```python
from build123d import *

# Parameters (mm, degrees)
F0_R      = 156.7807212082
F2_DEPTH  = 723.103761673
F4_DEPTH  = 289.7283732891
F5_DEPTH  = 25.4
F5_FACE_R = 156.7807212082


with BuildPart() as f2:
    # F0 (on Top) → F2 (new body)
    with BuildSketch(Plane.XY):
        Circle(F0_R)
    extrude(amount=F2_DEPTH)

    # F4 (add): a face of the model
    f4_faces = [f2.faces().sort_by_distance(p)[0] for p in [
        (0, 0, 0),
    ]]
    extrude(f4_faces, amount=F4_DEPTH)

    # F5 (add): a face of the model
    f5_faces = [f2.faces().sort_by_distance(p)[0] for p in [
        (0, 0, -289.7283732891),
    ]]
    extrude(f5_faces, amount=F5_DEPTH)

    # F5_face (on face) → F6 section 0
    with BuildSketch(Plane(origin=(0, 0, -315.1283732891), x_dir=(1, 0, 0), z_dir=(0, 0, -1)), mode=Mode.PRIVATE) as f6_s0:
        Circle(F5_FACE_R)
    loft([f6_s0.sketch, Vertex(0, 0, -691.5580034256)])


solid = f2.part
```
Geometry check sheet. Reference: the model listing, model coordinates, mm. Give positions to 0.01 mm unless a question says otherwise; leave off trailing zeros. Loops run counter-clockwise (first coordinate to the right, second up) from the corner with the lowest first, then second, coordinate; pieces in that order, holes last. Notation, with made-up numbers: M 64,74 L 80,74 A19 ccw 80,111 Z; hole C 64,20 d8. An arc over 180 degrees is marked long. Answer as CSV lines item,"result".
Item 1: Cross-section at B-B on z = -486.5. Record the cut outline in (x, y).
Values:
outline,"C 0,0 d170.81"
Item 2: Depth check by flat-ended pin: P1, Ø1.5, axis at y = -85, z = 559.5, coming from the -X side; P2, Ø3, axis at y = 85, z = -44.5, coming from the -X side; P3, Ø3, axis at y = 21, z = 47.5, coming from the +X side. Enter the tip coordinate at first touch or a pass-through.
Values:
P1,"stops at x = -132.22"
P2,"stops at x = -132.69"
P3,"stops at x = 155.56"
Item 3: Material ranges on line 1 (Z direction, x = 43, y = 86); line 2 (Z direction, x = -23.5, y = -53); line 3 (Y direction, x = -45.5, z = -46), recorded low to high.
Values:
line 1,"z = -460.7 to 723.1"
line 2,"z = -552.36 to 723.1"
line 3,"y = -150.03 to 150.03"
Item 4: Cross-section at A-A on z = -1.5. Record the cut outline in (x, y).
Values:
outline,"C 0,0 d313.56"
